The drawing under review shows one solid part. Ordinate dimensions are in mm from its lowest x, y, z. Round coordinates to 2 decimals unless told otherwise and drop trailing zeros. Order: outer loops, then holes, each group sorted by start corner. A loop starts at its lowest first (then second) coordinate and runs counter-clockwise, first axis right, second up. Notation, with made-up numbers: M -14.5,-30.5 L 4.5,-30.5 A18 cw 4.5,-25.5 Z; hole C 39.25,32 d11. An arc over 180 degrees is marked long. Use a Markdown table: item, result.
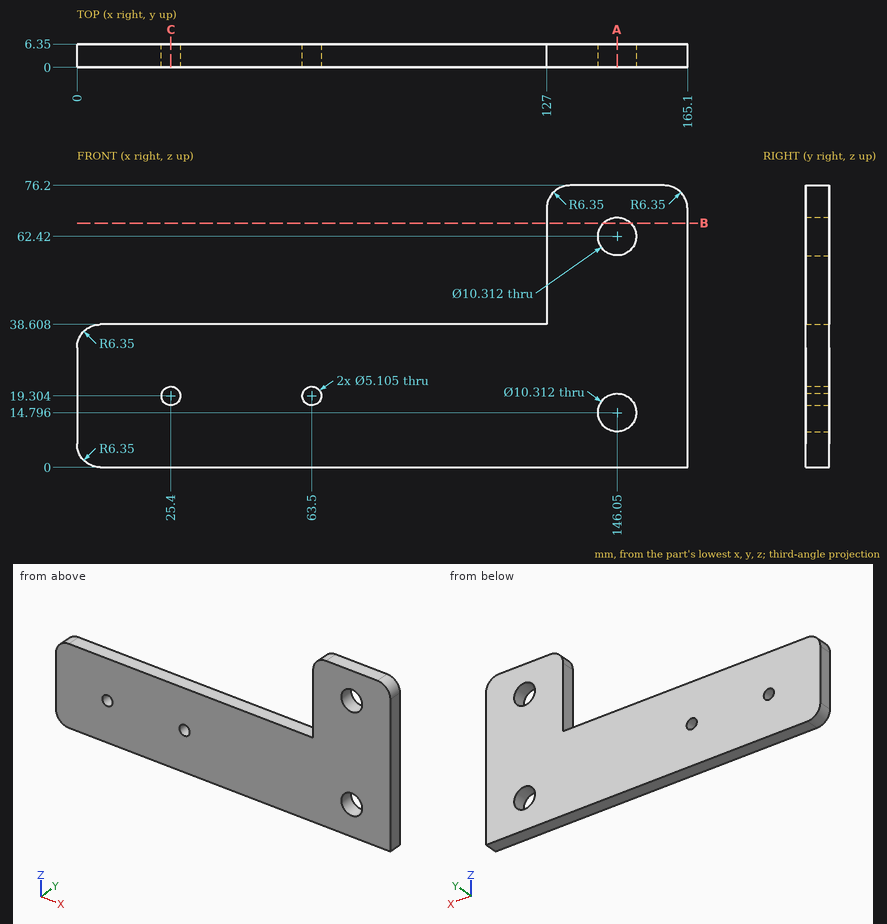
Q1. Clearance check with flat-ended pins moving along their axes: pin 1 (8 mm diameter, centred on x = 146.05, z = 14.8, fed in from +Y); pin 2 (2 mm diameter, centred on x = 41, y = 3.5, fed in from +Z). State where each tip first meets the part, or that it passes through.
Determined:
| item | result |
|---|---|
| pin 1 | passes through |
| pin 2 | stops at z = 38.61 |
Q2. Add section A-A (x = 146.05). Give the number of separate pieces and of enclosed holes in the cut face, then the cut area to 3 significant figures.
Determined:
| item | result |
|---|---|
| separate pieces | 3 |
| enclosed holes | 0 |
| area | 353 mm^2 |
Q3. Wall thickness on line 1 along Z through (x, y) = (146.05, 2.5) (1 decimal); line 2 along X through (y, z) = (3.75, 62); line 3 along Z through (x, y) = (63.5, 1.5): over which ranges is each line inside the solid? List them lowest first. Write a range as [from, to].
Determined:
| item | result |
|---|---|
| line 1 | z = [0, 9.6], [20, 57.3], [67.6, 76.2] |
| line 2 | x = [127, 140.91], [151.19, 165.1] |
| line 3 | z = [0, 16.75], [21.86, 38.61] |
Q4. Add section C-C (x = 25.4). Write out the cut boundary in (y, z).
Determined:
| item | result |
|---|---|
| outline | M 0,0 L 6.35,0 L 6.35,16.75 L 0,16.75 Z; M 0,21.86 L 6.35,21.86 L 6.35,38.61 L 0,38.61 Z |
Q5. Add section B-B (z = 66). Write out the cut boundary in (x, y).
Determined:
| item | result |
|---|---|
| outline | M 127,0 L 142.34,0 L 142.34,6.35 L 127,6.35 Z; M 149.76,0 L 165.1,0 L 165.1,6.35 L 149.76,6.35 Z |
